The model under review builds one solid part; all positions refer to its coordinate system, in mm. Coordinates: 2 decimals unless noted, no trailing zeros. Write each loop counter-clockwise with the first axis right and the second up, starting at its lowest first coordinate (ties: lowest second). Pieces come first, ordered by that corner, then holes. Notation, with made-up numbers: (-34, 24) -> (8, 24) arc R14 ccw to (8, 29) -> close; hole circle Ø7 at (75, 77.5). An arc over 180 degrees is marked (long way). Write each question's results on one line, items separated by ' | '.
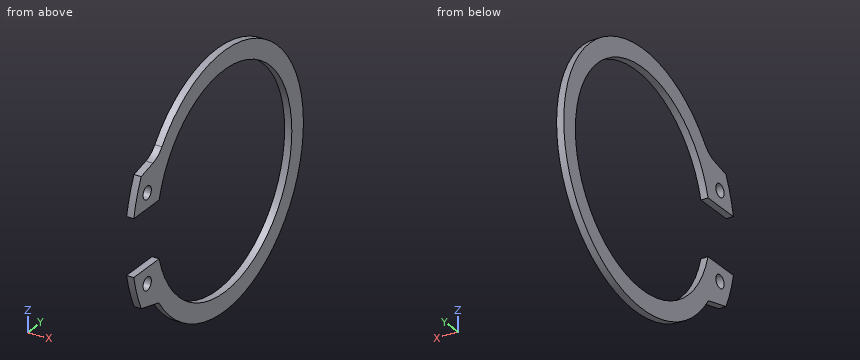
```python
from build123d import *

# Parameters (mm, degrees)
ESQUISSE1_R        = 2.5
BOSS_EXTRU_1_DEPTH = 2.75


with BuildPart() as part:
    # Esquisse1 → Boss.-Extru.1 (new body)
    with BuildSketch(Plane(origin=(0, 0, 0), x_dir=(0, 0, -1), z_dir=(1, 0, 0))):
        with BuildLine():
            ThreePointArc((-25.916566448, -43.057123424), (-27.227783117, -40.022676723), (-29.456638889, -37.581497115))
            ThreePointArc((-29.456638889, -37.581497115), (1.652244952, 47.721405958), (26.786870524, -39.528800482))
            Line((26.786870524, -39.528800482), (24.173691188, -50.122960456))
            ThreePointArc((24.173691188, -50.122960456), (17.612583106, -52.787076324), (10.766267997, -54.596391675))
            Line((10.766267997, -54.596391675), (10.766267997, -39.302035233))
            ThreePointArc((10.766267997, -39.302035233), (0, 40.75), (-10.766267997, -39.302035233))
            Line((-10.766267997, -39.302035233), (-10.766267997, -54.596391675))
            ThreePointArc((-10.766267997, -54.596391675), (-17.612583106, -52.787076324), (-24.173691188, -50.122960456))
            Line((-24.173691188, -50.122960456), (-25.916566448, -43.057123424))
        make_face()
        with Locations((-16.653577526, -46.504624781)):
            Circle(ESQUISSE1_R, mode=Mode.SUBTRACT)
        with Locations((16.653577526, -46.504624781)):
            Circle(ESQUISSE1_R, mode=Mode.SUBTRACT)
    extrude(amount=BOSS_EXTRU_1_DEPTH)


solid = part.part
```
Q1. Add section B-B (z = -12.5). Write out the cut boundary in (x, y), plus the area to 3 significant figures.
Solution:
outline: (0, -54.23) -> (2.75, -54.23) -> (2.75, -38.79) -> (0, -38.79) -> close; (0, 38.79) -> (2.75, 38.79) -> (2.75, 46.08) -> (0, 46.08) -> close | area: 62.5 mm²
Q2. For line 1 (Y direction, x = 1.65, z = -16.5); line 2 (Y direction, x = 1.9, z = 0); line 3 (Z direction, x = 0.8, y = -14), list the stretches that pass through material, from the lowest coordinate up. Write a range as from..to.
Solution:
line 1: -53.15..-49, -44.01..-37.26, 37.26..44.81 | line 2: 40.75..47.75 | line 3: -45.65..-38.27, 38.27..45.65
Q3. Add section D-D (z = 0). Write out the cut boundary in (x, y), plus the area to 4 significant figures.
Solution:
outline: (0, 40.75) -> (2.75, 40.75) -> (2.75, 47.75) -> (0, 47.75) -> close | area: 19.25 mm²
Q4. Add section C-C (x = 1.6). Write out the cut boundary in (y, z).
Solution:
outline: (-54.6, -10.77) arc R55.65 ccw to (-50.12, -24.17) -> (-39.53, -26.79) arc R47.75 ccw (long way) to (-37.58, 29.46) arc R10 cw to (-43.06, 25.92) -> (-50.12, 24.17) arc R55.65 ccw to (-54.6, 10.77) -> (-39.3, 10.77) arc R40.75 cw (long way) to (-39.3, -10.77) -> close; hole circle Ø5 at (-46.5, -16.65); hole circle Ø5 at (-46.5, 16.65)
Q5. Clearance check with flat-ended pins moving along their axes: P1, Ø12, axis at y = 3.5, z = -34, coming from the +X side; P2, Ø1.5, axis at x = 2.5, y = 9.5, coming from the -Z side; P3, Ø1, axis at x = 2.5, z = 12.5, coming from the -Y side; P4, Ø0.8, axis at x = 0.5, y = -46, coming from the -Z side. State where each tip first meets the part, or that it passes through.
Solution:
P1: through | P2: z = -46.94 | P3: y = -54.34 | P4: z = -25.29
Q6. Add section A-A (y = 0). Write out the cut boundary in (x, z), plus the area to 3 significant figures.
Solution:
outline: (0, -47.75) -> (2.75, -47.75) -> (2.75, -40.75) -> (0, -40.75) -> close; (0, 40.75) -> (2.75, 40.75) -> (2.75, 47.75) -> (0, 47.75) -> close | area: 38.5 mm²
